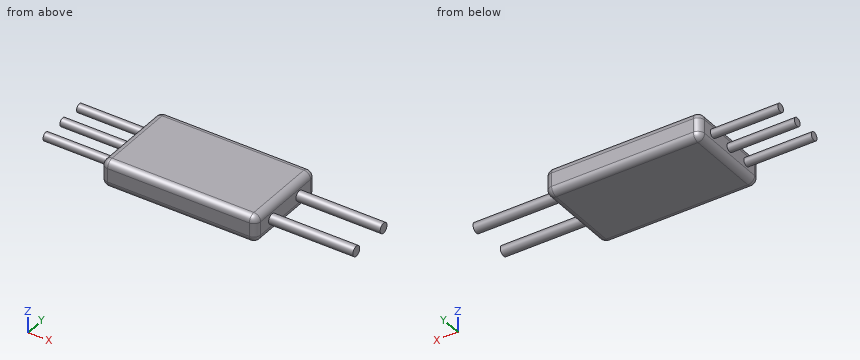
Autodesk Inventor part; units mm, degrees
ref_plane "YZ Plane" through (0, 0, 0) normal (1, 0, 0) x (0, 1, 0)
ref_plane "XZ Plane" through (0, 0, 0) normal (0, 1, 0) x (-1, 0, 0)
ref_plane "XY Plane" through (0, 0, 0) normal (0, 0, 1) x (1, 0, 0)
sketch "Sketch1" plane through (0, 0, 0) normal (0, 0, 1) x (1, 0, 0)
  line L0 (0, 0) -> (-46, 0)
  line L1 (-46, 0) -> (-46, 26)
  line L2 (-46, 26) -> (0, 26)
  line L3 (0, 26) -> (0, 0)
  dimension "d0" = 46
  dimension "d1" = 26
extrude "Extrusion1" add sketch "Sketch1" along normal blind 8
fillet "Fillet1" radius 2 12 edges at (-23, 26, 8) (-46, 13, 8) (-46, 26, 4) (0, 13, 8) (-23, 0, 8) (0, 26, 4) (0, 13, 0) (0, 0, 4) (-23, 0, 0) (-46, 0, 4) (-46, 13, 0) (-23, 26, 0)
sketch "Sketch2" plane through (0, 2, 6) normal (1, 0, 0) x (0, 0, -1)
  circle A0 centre (2, 17) radius 1.5
  line L0 (0, 0) -> (0, 22)
  line L1 (0, 22) -> (4, 22)
  line L2 (4, 22) -> (4, 0)
  line L3 (4, 0) -> (0, 0)
  circle A1 centre (2, 5) radius 1.5
  line L4 (2, 26.4217) -> (2, -4.8985)
  point P0 (6, -2)
  dimension "d5" = 3
  dimension "d6" = 3
  dimension "d7" = 5
  dimension "d8" = 5
extrude "Extrusion2" add sketch "Sketch2" along normal blind 25 contours A0 L4 | L4 A0 | L4 A1 | A1 L4
sketch "Sketch3" plane through (-46, 2, 2) normal (-1, 0, 0) x (0, 0, 1)
  line L0 (4, 22) -> (4, 0)
  line L1 (0, 22) -> (4, 22)
  line L2 (0, 22) -> (4, 22)
  line L3 (0, 0) -> (0, 22)
  line L4 (4, 0) -> (0, 0)
  line L5 (4, 22) -> (4, 0)
  circle A0 centre (2, 18.2633) radius 1.25
  circle A1 centre (2, 10.9374) radius 1.25
  circle A2 centre (2, 3.4881) radius 1.25
  line L6 (2, 27.5735) -> (2, -5.6987)
  point P0 (-2, -2)
  dimension "d11" = 2.5
  dimension "d12" = 2.5
  dimension "d13" = 2.5
extrude "Extrusion3" add sketch "Sketch3" along normal blind 20 contours L6 A0 | A0 L6 | L6 A2 | A2 L6 | L6 A1 | A1 L6
properties part number "Esc_BlHeli_30A"
Input: part model. Units: mm. Frame: model coordinates. Coordinates: 2 decimals unless noted, no trailing zeros. Loops run counter-clockwise (first coordinate to the right, second up) from the corner with the lowest first, then second, coordinate; pieces in that order, holes last. Notation, with made-up numbers: (-36, 27) -> (1, 27) arc R15 ccw to (1, 44) -> close; hole circle Ø5 at (-18, -24.5). An arc over 180 degrees is marked (long way). One line per item, written item: value.
(1) Ray query, line 1 along Y through (x, z) = (-51.5, 3.75); line 2 along Y through (x, z) = (-57, 4.5); line 3 along Y through (x, z) = (-17.5, 1.75). Return the intervals inside material, ascending.
Answer below:
line 1: y = 4.26 to 6.71, 11.71 to 14.16, 19.04 to 21.49
line 2: y = 4.34 to 6.63, 11.79 to 14.08, 19.12 to 21.41
line 3: y = 0.02 to 25.98
(2) Cut plane B-B (x = -40.5). Output: boundary loops of the cut face in (y, z), then the cut area to 3 significant figures.
Answer below:
outline: (0, 2) arc R2 ccw to (2, 0) -> (24, 0) arc R2 ccw to (26, 2) -> (26, 6) arc R2 ccw to (24, 8) -> (2, 8) arc R2 ccw to (0, 6) -> close
area: 205 mm2
(3) Pin query (flat end, axial travel): pin 1 Ø3 at (x, z) = (-54, 6.5) entering from -Y; pin 2 Ø4 at (y, z) = (16, 4) entering from +X; pin 3 Ø1.5 at (x, z) = (8, 2.5) entering from -Y; pin 4 Ø2 at (y, z) = (15.5, 4.5) entering from -X. Return the tip coordinate at first contact, or that it passes through.
Answer below:
pin 1: stops at y = 4.74
pin 2: stops at x = 25
pin 3: stops at y = 5.7
pin 4: stops at x = -46
(4) Cut plane C-C (x = 5.5). Output: boundary loops of the cut face in (y, z).
Answer below:
outline: circle Ø3 at (7, 4); circle Ø3 at (19, 4)
(5) Cut plane A-A (z = 4). Output: boundary loops of the cut face in (x, y).
Answer below:
outline: (-66, 4.24) -> (-46, 4.24) -> (-46, 2) arc R2 ccw to (-44, 0) -> (-2, 0) arc R2 ccw to (0, 2) -> (0, 5.5) -> (25, 5.5) -> (25, 8.5) -> (0, 8.5) -> (0, 17.5) -> (25, 17.5) -> (25, 20.5) -> (0, 20.5) -> (0, 24) arc R2 ccw to (-2, 26) -> (-44, 26) arc R2 ccw to (-46, 24) -> (-46, 21.51) -> (-66, 21.51) -> (-66, 19.01) -> (-46, 19.01) -> (-46, 14.19) -> (-66, 14.19) -> (-66, 11.69) -> (-46, 11.69) -> (-46, 6.74) -> (-66, 6.74) -> close
